from build123d import *

# Parameters (mm, degrees)
SKETCH2_R               = 33.1665
SKETCH2_R_2             = 11.1
BOSS_EXTRUDE1_DEPTH     = 7.175
SKETCH2_5_R             = 34.6665
SKETCH2_5_R_2           = 33.1665
BOSS_EXTRUDE2_DEPTH     = 12.175
CIRPATTERN1_COUNT       = 3
CUT_EXTRUDE3_REACH      = 85.886
CUT_EXTRUDE3_END_RADIUS = 11.1
SKETCH5_R               = 1.5
CIRPATTERN2_COUNT       = 3


with BuildPart() as part:
    # Sketch2 → Boss-Extrude1 (new body)
    with BuildSketch(Plane(origin=(0, 0, 0), x_dir=(1, 0, 0), z_dir=(0, 1, 0))):
        with Locations(Location((0, 0, 0), (0, 0, 270))):
            Circle(SKETCH2_R)
        with Locations(Location((0, 0, 0), (0, 0, 270))):
            Circle(SKETCH2_R_2, mode=Mode.SUBTRACT)
    extrude(amount=BOSS_EXTRUDE1_DEPTH)

    # Sketch2_5 → Boss-Extrude2 (add)
    with BuildSketch(Plane(origin=(0, 0, 0), x_dir=(1, 0, 0), z_dir=(0, 1, 0))):
        with Locations(Location((0, 0, 0), (0, 0, 270))):
            Circle(SKETCH2_5_R)
        with Locations(Location((0, 0, 0), (0, 0, 270))):
            Circle(SKETCH2_5_R_2, mode=Mode.SUBTRACT)
    extrude(amount=BOSS_EXTRUDE2_DEPTH)

    # Sketch3 → Cut-Revolve1 (revolve, cut)
    with BuildSketch(Plane.XZ):
        with BuildLine():
            Line((2.5019, 18), (-2.5019, 18))
            ThreePointArc((-2.5019, 18), (0, 15.4981), (2.5019, 18))
        make_face()
    cut_revolve1 = revolve(axis=Axis((3.292813159, 0, 18), (-1, 0, 0)), mode=Mode.SUBTRACT)

    # CirPattern1: Cut-Revolve1 ×3 about axis
    cirpattern1_axis = Axis((0, 0, 0), (0, 1, 0))
    for i in range(1, CIRPATTERN1_COUNT):
        add(cut_revolve1.rotate(cirpattern1_axis, i * 360 / CIRPATTERN1_COUNT), mode=Mode.SUBTRACT)

    # Cut-Extrude3: up to this cylinder (the profile starts outside it)
    cut_extrude3_end = Plane(origin=(0, 3.5875, 0), z_dir=(0, -1, 0)) * Cylinder(CUT_EXTRUDE3_END_RADIUS, 194.972, mode=Mode.PRIVATE)
    # Sketch5 → Cut-Extrude3 (cut, up to the surface)
    with BuildSketch(Plane(origin=(30.02206966, 0, 17.33325), x_dir=(0.4999999999999922, 0, -0.8660254037844431), z_dir=(0.8660254037844431, 0, 0.4999999999999922)), mode=Mode.PRIVATE) as cut_extrude3_sk1:
        with Locations((0, 3.5875)):
            Circle(SKETCH5_R)
    cut_extrude3_tool1 = extrude(cut_extrude3_sk1.sketch, amount=-CUT_EXTRUDE3_REACH, mode=Mode.PRIVATE) - cut_extrude3_end
    cut_extrude3 = cut_extrude3_tool1.solids().sort_by_distance((30.02207, 3.5875, 17.33325))[0]
    add(cut_extrude3, mode=Mode.SUBTRACT)

    # CirPattern2: Cut-Extrude3 ×3 about axis
    cirpattern2_axis = Axis((0, 12.175, 0), (0, -1, 0))
    for i in range(1, CIRPATTERN2_COUNT):
        add(cut_extrude3.rotate(cirpattern2_axis, i * 360 / CIRPATTERN2_COUNT), mode=Mode.SUBTRACT)


solid = part.part
Check sheet for the modelled part. Datum: model origin and axes. Units: mm. A direction names the side the tool comes from. Give positions to 0.01 mm unless a question says otherwise; leave off trailing zeros. Write each loop counter-clockwise with the first axis right and the second up, starting at its lowest first coordinate (ties: lowest second). Pieces come first, ordered by that corner, then holes. Notation, with made-up numbers: (-38, -15.5) -> (-12, -15.5) arc R16 ccw to (-12, -9.5) -> close; hole circle Ø5 at (71, 2). An arc over 180 degrees is marked (long way). Use one line per item in the form item = value. Start each with the question number.
1. Thickness scan on line 1 along X through (y, z) = (4.5, 0); line 2 along Z through (x, y) = (18, 9.75). Record the ranges inside material, lowest first. Write a range as from..to.
2. Section check B-B (z = 0). Record the cut outline in (x, y) (1 decimal), and give its area (3 significant figures).
3. Go/stop test with flat-tipped pins: P1, Ø5, axis at y = 7.5, z = 16, coming from the -X side; P2, Ø5, axis at x = 14, y = 2, coming from the +Z side; P3, Ø3, axis at x = -12, z = -11.5, coming from the +Y side (3 decimals). Record where each tip stops, or that it passes through.
4. Section check C-C (x = 7.5). Record the cut outline in (y, z) (3 decimals).
5. Section check A-A (x = 0). Record the cut outline in (y, z) (1 decimal).
6. Access from +Z, -Z, +X, -X, +Y, -Y to the whole of each face (thin tool, end or side, straight path). Record for faces 4 (the flat face through (-14, 7.175, 0)), 5 (the cylindrical face through (1.19, 2.675, -22.996)), 6 (the cylindrical face through (19.32, 2.675, 12.529)).
7. Mould release check, pull along Z, two halves, no side actions. Record for faces 1 (the flat face through (8, 0, -8)), 2 (the cylindrical face through (7.502, 3.537, -8.181)), 3 (the cylindrical face through (-21.094, 6.002, -27.51)): pulls with the +Z half, pulls with the -Z half, needs draft (parallel to the pull), parting line crosses it, or undercut.
Conclusion:
q1.line_1 = -34.67..-11.1, 11.1..34.67
q1.line_2 = -29.63..-27.86, 27.86..29.63
q2.outline = (-34.7, 0) -> (-11.1, 0) -> (-11.1, 7.2) -> (-33.2, 7.2) -> (-33.2, 12.2) -> (-34.7, 12.2) -> close; (11.1, 0) -> (34.7, 0) -> (34.7, 12.2) -> (33.2, 12.2) -> (33.2, 7.2) -> (11.1, 7.2) -> close
q2.area = 353 mm²
q3.P1 = -31.93
q3.P2 = 32.7
q3.P3 = 7.175
q4.outline = (0, -33.845) -> (12.175, -33.845) -> (12.175, -32.307) -> (7.175, -32.307) -> (7.175, -8.183) -> (0, -8.183) -> close; (0, 8.183) -> (7.175, 8.183) -> (7.175, 32.307) -> (12.175, 32.307) -> (12.175, 33.845) -> (0, 33.845) -> close
q5.outline = (0, -34.7) -> (2.1, -34.7) -> (2.1, -11.1) -> (0, -11.1) -> close; (0, 11.1) -> (7.2, 11.1) -> (7.2, 33.2) -> (12.2, 33.2) -> (12.2, 34.7) -> (0, 34.7) -> (0, 20.5) arc R2.5 cw to (0, 15.5) -> close; (5.1, -34.7) -> (12.2, -34.7) -> (12.2, -33.2) -> (7.2, -33.2) -> (7.2, -11.1) -> (5.1, -11.1) -> close
q6.face_4 = +Y
q6.face_5 = -Z
q6.face_6 = none
q7.face_1 = needs draft
q7.face_2 = undercut
q7.face_3 = parting line crosses it
